Input: part model. Units: mm. Frame: model coordinates. A direction names the side the tool comes from. Round coordinates to 2 decimals unless told otherwise and drop trailing zeros. Loops run counter-clockwise (first coordinate to the right, second up) from the corner with the lowest first, then second, coordinate; pieces in that order, holes last. Notation, with made-up numbers: (1, 20.5) -> (6, 20.5) arc R16 cw to (6, 29.5) -> close; hole circle Ø5 at (2, -26.5). An arc over 180 degrees is marked (long way). Answer as a JSON object with one key per item and string values. Group by question number.
Item 1: Section query C-C on x = -2.5. Return loops of the section in (y, z), and give its area (3 significant figures).
Item 2: Section query D-D on y = -8.5. Return loops of the section in (x, z), and give its area (3 significant figures).
Item 3: Section query B-B on x = -11. Return loops of the section in (y, z), and give its area (3 significant figures).
Item 4: Section query A-A on z = 18.75. Return loops of the section in (x, y), and give its area (3 significant figures).
Item 5: Draft query along Z for faces 1 (the cylindrical face through (-1.52, -14.96, 21.66)), 2 (the flat face through (-2.507, -5.617, 6.095)), 3 (the cylindrical face through (-21.9, -7.7, 0)), 4 (the cylindrical face through (-1, -7.6, 24.9)). Return one class per face: released by +Z, released by -Z, zero draft, split by the parting line, or undercut.
Item 6: Material intervals for line 1 (X direction, y = -12.5, z = 18); line 2 (Z direction, x = -11.75, y = -3.75); line 3 (Y direction, x = -1, z = 18.5), sorted ascending. Write a range as [from, to].
Item 7: Set-up query: faces 5 (the flat face through (-15, -10.12, 0)), 6 (the flat face through (-2.5, -3.67, 16.1)), 7 (the flat face through (-22.837, -9.567, 2.014)), 8 (the flat face through (-1, -10.12, 16)). Return all of +Z, -Z, +X, -X, +Y, -Y with unobstructed straight access to the full face (end or side cutting, diameter ignored); none if empty.
Item 8: Pin query (flat end, axial travel): pin 1 (1.6 mm diameter, centred on x = -18, z = 1.5, fed in from +Y); pin 2 (5 mm diameter, centred on y = -2, z = 4, fed in from -X); pin 3 (6.5 mm diameter, centred on y = -7.5, z = 11.5, fed in from -X); pin 4 (2 mm diameter, centred on y = -10.5, z = 6, fed in from -X). Return the tip coordinate at first contact, or that it passes through.
from build123d import *

# Parameters (mm, degrees)
F1_DEPTH    = 15.24
F3_DEPTH    = 1
F4_DEPTH    = 3
F6_DEPTH    = 2
F7_DEPTH    = 4
F8_SIZE2    = 6.6595190754
F8_SIZE     = 5.588
F9_T1_DEPTH = 11.189330271
F9_T3_DEPTH = 13.4919223085
F10_R       = 7.61999


# Not quite as in the source:
# - a fillet or chamfer that OpenCascade refuses, or shapes differently, is made with other operations: its cross-section is extruded or revolved along the edge and cut away or added
# - a fillet or chamfer is up to 0.001 mm smaller than in the source, because OpenCascade refuses the exact size


with BuildPart() as f1:
    # F0 (on Front) → F1 (new body)
    with BuildSketch(Plane.XZ):
        with BuildLine():
            ThreePointArc((-3, 4.5), (-3.4393398282, 3.4393398282), (-4.5, 3))
            Line((-4.5, 3), (-25.4, 3))
            Line((-25.4, 3), (-25.4, -1))
            Line((-25.4, -1), (-1.5, -1))
            ThreePointArc((-1.5, -1), (-0.4393398282, -0.5606601718), (0, 0.5))
            Line((0, 0.5), (0, 28.4))
            Line((0, 28.4), (-3, 28.4))
            Line((-3, 28.4), (-3, 4.5))
        make_face()
    extrude(amount=F1_DEPTH)

    # F2 (on face) → F3 (cut)
    with BuildSketch(Plane(origin=(-3, 0, 0), x_dir=(0, -1, 0), z_dir=(-1, 0, 0))):
        Polygon((11.57, 20.1194664367), (11.57, 22.4), (11.57, 24.6805335633), (7.62, 26.9610671266), (3.67, 24.6805335633), (3.67, 22.4), (3.67, 20.1194664367), (3.67, 11.7805335633), (3.67, 9.5), (3.67, 7.2194664367), (7.62, 4.9389328734), (11.57, 7.2194664367), (11.57, 9.5), (11.57, 11.7805335633), align=None)
        with BuildLine():
            Line((5.12, 9.5), (5.12, 22.4))
            ThreePointArc((5.12, 22.4), (7.62, 24.9), (10.12, 22.4))
            Line((10.12, 22.4), (10.12, 9.5))
            ThreePointArc((10.12, 9.5), (7.62, 7), (5.12, 9.5))
        make_face(mode=Mode.SUBTRACT)
    extrude(amount=-F3_DEPTH, mode=Mode.SUBTRACT)

    # F4 (cut, through all): a face of the model
    f4_faces = [f1.faces().sort_by_distance(p)[0] for p in [
        (-3, -7.62, 15.95),
    ]]
    extrude(f4_faces, amount=-F4_DEPTH, mode=Mode.SUBTRACT)

    # F5 (on face) → F6 (cut)
    with BuildSketch(Plane.XY.offset(3)):
        Polygon((-21.6805335633, -11.57), (-7.9645335633, -11.57), (-5.938922, -7.52), (-7.9645335633, -3.67), (-21.6805335633, -3.67), (-23.9610671266, -7.62), align=None)
        with BuildLine():
            Line((-10.5, -10.12), (-19.4, -10.12))
            ThreePointArc((-19.4, -10.12), (-21.9, -7.62), (-19.4, -5.12))
            Line((-19.4, -5.12), (-10.5, -5.12))
            ThreePointArc((-10.5, -5.12), (-8, -7.62), (-10.5, -10.12))
        make_face(mode=Mode.SUBTRACT)
    extrude(amount=-F6_DEPTH, mode=Mode.SUBTRACT)

    # F7 (cut, through all): a face of the model
    f7_faces = [f1.faces().sort_by_distance(p)[0] for p in [
        (-14.95, -7.62, 3),
    ]]
    extrude(f7_faces, amount=-F7_DEPTH, mode=Mode.SUBTRACT)

    # F8
    f8_edges = [f1.edges().sort_by_distance(p)[0] for p in [
        (-1.5, -15.24, 28.4),
        (-1.5, 0, 28.4),
    ]]
    f8_side = f1.faces().sort_by_distance((-1.5, -7.62, 28.4))[0]
    chamfer(f8_edges, length=F8_SIZE, length2=F8_SIZE2, reference=f8_side)

    # F9: fillet of radius 4.5 on 4 edges, made by hand

    # F9_s2 → F9_t1 (cut)
    with BuildSketch(Plane.YZ.offset(-7.0946651355)):
        with BuildLine():
            ThreePointArc((-14.187199994, 22.995159114), (-14.9686167935, 21.6417055154), (-15.24, 20.1026148704))
            Line((-15.24, 20.1026148704), (-15.24, 21.7404809246))
            Line((-15.24, 21.7404809246), (-14.187199994, 22.995159114))
        make_face()
        with BuildLine():
            ThreePointArc((-1.052800006, 22.995159114), (-0.2713832065, 21.6417055154), (0, 20.1026148704))
            Line((0, 20.1026148704), (0, 21.7404809246))
            Line((0, 21.7404809246), (-1.052800006, 22.995159114))
        make_face()
    extrude(amount=F9_T1_DEPTH, mode=Mode.SUBTRACT)

    # F9_s4 → F9_t3 (cut)
    with BuildSketch(Plane.YZ.offset(-8.2459611542)):
        with BuildLine():
            ThreePointArc((-7.5536155383, 28.4), (-9.4553977161, 27.9783850417), (-11.0008155323, 26.7925442436))
            Line((-11.0008155323, 26.7925442436), (-9.652, 28.4))
            Line((-9.652, 28.4), (-7.5536155383, 28.4))
        make_face()
        with BuildLine():
            ThreePointArc((-7.6863844617, 28.4), (-5.7846022839, 27.9783850417), (-4.2391844677, 26.7925442436))
            Line((-4.2391844677, 26.7925442436), (-5.588, 28.4))
            Line((-5.588, 28.4), (-7.6863844617, 28.4))
        make_face()
    extrude(amount=F9_T3_DEPTH, mode=Mode.SUBTRACT)

    # F10 (radius 7.62 in the source; OpenCascade refuses exactly that, so slightly less here)
    f10_edges = [f1.edges().sort_by_distance(p)[0] for p in [
        (-25.4, -15.24, 1),
        (-25.4, 0, 1),
    ]]
    fillet(f10_edges, radius=F10_R)


solid = f1.part
Solved:
{
 "1": {"outline": "(-15.24, -1) -> (0, -1) -> (0, 20.1) arc R4.5 ccw to (-1.05, 23) -> (-4.24, 26.79) arc R4.5 ccw to (-7.62, 28.4) arc R4.5 ccw to (-11, 26.79) -> (-14.19, 23) arc R4.5 ccw to (-15.24, 20.1) -> close; hole (-11.57, 7.22) -> (-7.62, 4.94) -> (-3.67, 7.22) -> (-3.67, 24.68) -> (-7.62, 26.96) -> (-11.57, 24.68) -> close", "area": "253 mm²"},
 "2": {"outline": "(-25.35, -1) -> (-21.74, -1) -> (-21.74, 1) -> (-23.45, 1) -> (-23.45, 3) -> (-25.35, 3) -> close; (-8.16, -1) -> (-1.5, -1) arc R1.5 ccw to (0, 0.5) -> (0, 7.16) -> (-2, 7.16) -> (-2, 5.45) -> (-3, 5.45) -> (-3, 4.5) arc R1.5 cw to (-4.5, 3) -> (-6.43, 3) -> (-6.43, 1) -> (-8.16, 1) -> close; (-3, 26.45) -> (-2, 26.45) -> (-2, 24.74) -> (0, 24.74) -> (0, 28.3) -> (-3, 28.3) -> close", "area": "59.9 mm²"},
 "3": {"outline": "(-15.24, -1) -> (-10.12, -1) -> (-10.12, 1) -> (-11.57, 1) -> (-11.57, 3) -> (-15.24, 3) -> close; (-5.12, -1) -> (0, -1) -> (0, 3) -> (-3.67, 3) -> (-3.67, 1) -> (-5.12, 1) -> close", "area": "35.2 mm²"},
 "4": {"outline": "(-3, -15.24) -> (0, -15.24) -> (0, -10.12) -> (-2, -10.12) -> (-2, -11.57) -> (-3, -11.57) -> close; (-3, -3.67) -> (-2, -3.67) -> (-2, -5.12) -> (0, -5.12) -> (0, 0) -> (-3, 0) -> close", "area": "27.8 mm²"},
 "5": {"face 1": "released by +Z", "face 2": "undercut", "face 3": "zero draft", "face 4": "undercut"},
 "6": {"line 1": "[-3, 0]", "line 2": "[-1, 1]", "line 3": "[-15.24, -10.12], [-5.12, 0]"},
 "7": {"face 5": "+Z, -Z", "face 6": "-X", "face 7": "+Z", "face 8": "+X, -X"},
 "8": {"pin 1": "y = 0", "pin 2": "x = -24.63", "pin 3": "x = -2", "pin 4": "x = -3"}
}
